The model under review builds one solid part; all positions refer to its coordinate system, in mm. Face numbers are marked on the shaded views. Round coordinates to 2 decimals unless told otherwise and drop trailing zeros. Loops run counter-clockwise (first coordinate to the right, second up) from the corner with the lowest first, then second, coordinate; pieces in that order, holes last. Notation, with made-up numbers: M 13,-17 L 68,-17 A23 cw 68,2 Z; hole C -13.75,-36.75 d8. An arc over 180 degrees is marked long. One line per question, with ' | ' between items.
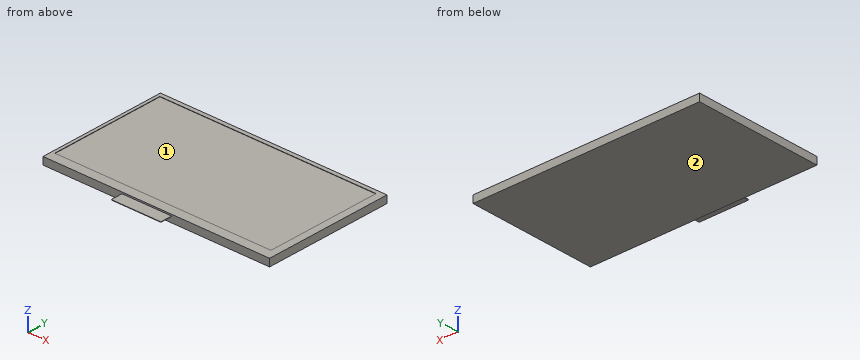
from build123d import *

# Parameters (mm, degrees)
SKETCH1_W           = 176.022
SKETCH1_H           = 100
SKETCH1_W_2         = 167.9702
SKETCH1_H_2         = 89.4844
BOSS_EXTRUDE1_DEPTH = 5.7
SKETCH1_3_W         = 167.9702
SKETCH1_3_H         = 89.4844
CUT_EXTRUDE1_DEPTH  = 0.254
BOSS_EXTRUDE2_START = -1.1684
SKETCH2_W           = 38.53942
SKETCH2_H           = 9.144
BOSS_EXTRUDE2_DEPTH = 0.3048


with BuildPart() as part:
    # Sketch1 → Boss-Extrude1 (new body)
    # profile 1 of 2: a face of its own
    with BuildSketch(Plane.XY):
        Rectangle(SKETCH1_W, SKETCH1_H)
        with Locations((-1.6383, 2.1336)):
            Rectangle(SKETCH1_W_2, SKETCH1_H_2, mode=Mode.SUBTRACT)
    # profile 2 of 2: a face of its own
    with BuildSketch(Plane.XY):
        with Locations((-1.6383, 2.1336)):
            Rectangle(SKETCH1_W_2, SKETCH1_H_2)
    extrude(amount=-BOSS_EXTRUDE1_DEPTH)

    # Sketch1_3 → Cut-Extrude1 (cut)
    with BuildSketch(Plane.XY):
        with Locations((-1.6383, 2.1336)):
            Rectangle(SKETCH1_3_W, SKETCH1_3_H)
    extrude(amount=-CUT_EXTRUDE1_DEPTH, mode=Mode.SUBTRACT)

    # Sketch2 → Boss-Extrude2 (add)
    with BuildSketch(Plane.XY.offset(BOSS_EXTRUDE2_START)):
        with Locations((-7.37489, -54.572)):
            Rectangle(SKETCH2_W, SKETCH2_H)
    extrude(amount=-BOSS_EXTRUDE2_DEPTH)


solid = part.part
1) Insertion check: P1, Ø3, axis at x = -35.5, z = -2.5, coming from the -Y side; P2, Ø6, axis at x = -42.5, y = 25, coming from the +Z side; P3, Ø2.5, axis at x = 1, y = -55, coming from the +Z side. Each pin has a flat end and moves straight along its axis. Give the tip position at first contact, or say it passes through.
Output values:
P1: stops at y = -50 | P2: stops at z = -0.25 | P3: stops at z = -1.17
2) For line 1 (Y direction, x = -21.5, z = -3.2); line 2 (Z direction, x = -43, y = 33); line 3 (Y direction, x = 39, z = -0.15), list the stretches that pass through material, from the lowest coordinate up.
Output values:
line 1: y = -50 to 50 | line 2: z = -5.7 to -0.25 | line 3: y = -50 to -42.61, 46.88 to 50
3) Add section C-C on z = -3.5. State the section outline as (x, y) points.
Output values:
outline: M -88.01,-50 L 88.01,-50 L 88.01,50 L -88.01,50 Z
4) Add section B-B on y = -18. State the section outline as (x, z) points.
Output values:
outline: M -88.01,-5.7 L 88.01,-5.7 L 88.01,0 L 82.35,0 L 82.35,-0.25 L -85.62,-0.25 L -85.62,0 L -88.01,0 Z
5) Mouldability with a two-part tool opening along Y and no side actions: class the marked faces 1 and 2 as +Y half, -Y half, draft (parallel to the pull), parting line (faces both ways), or undercut.
Output values:
face 1: undercut | face 2: draft
6) Add section A-A on x = -30.5. State the section outline as (y, z) points, then the cut area to 3 significant figures.
Output values:
outline: M -50,-5.7 L 50,-5.7 L 50,0 L 46.88,0 L 46.88,-0.25 L -42.61,-0.25 L -42.61,0 L -50,0 Z | area: 547 mm²
7) Add section D-D on x = -12. State the section outline as (y, z) points.
Output values:
outline: M -59.14,-1.47 L -50,-1.47 L -50,-5.7 L 50,-5.7 L 50,0 L 46.88,0 L 46.88,-0.25 L -42.61,-0.25 L -42.61,0 L -50,0 L -50,-1.17 L -59.14,-1.17 Z
